```python
from build123d import *

# Parameters (mm, degrees)
SKETCH1_R           = 1.65
BOSS_EXTRUDE1_DEPTH = 22.4
SKETCH2_R           = 3.05
CUT_EXTRUDE1_DEPTH  = 3
CUT_EXTRUDE2_REACH  = 81.517
SKETCH3_W           = 0.4
SKETCH3_H           = 22.4


with BuildPart() as part:
    # Sketch1 → Boss-Extrude1 (new body)
    with BuildSketch(Plane.XY):
        Polygon((0, 0), (-75, 0), (-75, 7.5), (-0.787017068, 10), (72.903367057, 19.140247432), (74.076625545, 11.732584878), align=None)
        with Locations((-0.235377287, 2.990752001)):
            Circle(SKETCH1_R, mode=Mode.SUBTRACT)
    extrude(amount=BOSS_EXTRUDE1_DEPTH)

    # Sketch2 → Cut-Extrude1 (cut)
    with BuildSketch(Plane(origin=(0, 0, 0), x_dir=(0.9876883405951377, 0.15643446504023117, 0), z_dir=(0.1564344650402312, -0.9876883405951378, 0))):
        with Locations((67, 14.7)):
            Circle(SKETCH2_R)
        with Locations((67, 7.7)):
            Circle(SKETCH2_R)
    cut_extrude1 = extrude(amount=-CUT_EXTRUDE1_DEPTH, mode=Mode.SUBTRACT)

    # Mirror1: Cut-Extrude1 across plane
    add(cut_extrude1.mirror(Plane(origin=(0, 0, 0), x_dir=(0, 0, 1), z_dir=(0.9969173337331281, 0.07845909572784505, 0))), mode=Mode.SUBTRACT)

    # Cut-Extrude2: up to this plane
    cut_extrude2_end = Plane(origin=(-0.773549976, 9.600226767, 22.4), z_dir=(0.03366773042207346, -0.9994330812656876, 0))
    # Sketch3 → Cut-Extrude2 (cut, up to the surface)
    with BuildSketch(Plane(origin=(-1.048316472, 13.320123716, 0), x_dir=(0.9969173337331281, 0.07845909572784511, 0), z_dir=(-0.07845909572784511, 0.9969173337331281, 0)), mode=Mode.PRIVATE) as cut_extrude2_sk1:
        with Locations((0, -11.2)):
            Rectangle(SKETCH3_W, SKETCH3_H)
    cut_extrude2_tool1 = split(extrude(cut_extrude2_sk1.sketch, amount=-CUT_EXTRUDE2_REACH, mode=Mode.PRIVATE), bisect_by=cut_extrude2_end, keep=Keep.BOTH, mode=Mode.PRIVATE)
    add(cut_extrude2_tool1.solids().sort_by_distance((-1.048316, 13.320124, 11.2))[0], mode=Mode.SUBTRACT)


solid = part.part
```
Read the model definition and answer for the solid it produces. Units are mm, in the model's axes. A direction names the side the tool comes from. Round coordinates to 2 decimals unless told otherwise and drop trailing zeros. Loops run counter-clockwise (first coordinate to the right, second up) from the corner with the lowest first, then second, coordinate; pieces in that order, holes last. Notation, with made-up numbers: (33.25, 41.25) -> (39.25, 41.25) arc R24 ccw to (39.25, 77.25) -> close; hole circle Ø8 at (22, -18). An arc over 180 degrees is marked (long way). One line per item, written item: value.
1) A cutting plane is placed at B-B (x = -67). Determine the outline of the cut face in (y, z), and give its area (3 significant figures).
Answer list:
outline: (0, 0) -> (7.77, 0) -> (7.77, 22.4) -> (0, 22.4) -> (0, 17.75) -> (3, 17.75) -> (3, 11.65) -> (0, 11.65) -> (0, 10.75) -> (3, 10.75) -> (3, 4.65) -> (0, 4.65) -> close
area: 137 mm²
2) A cutting plane is placed at C-C (z = 16.25). Determine the outline of the cut face in (x, y), and give its area (3 significant figures).
Answer list:
outline: (-75, 0) -> (-69.63, 0) -> (-69.63, 3) -> (-64.37, 3) -> (-64.37, 0) -> (0, 0) -> (63.58, 10.07) -> (63.11, 13.03) -> (68.3, 13.86) -> (68.77, 10.89) -> (74.08, 11.73) -> (72.9, 19.14) -> (-0.59, 10.02) -> (-0.56, 9.61) -> (-0.96, 9.59) -> (-0.99, 9.99) -> (-75, 7.5) -> close; hole circle Ø3.3 at (-0.24, 2.99)
area: 1,270 mm²
3) A cutting plane is placed at A-A (z = 7.7). Determine the outline of the cut face in (x, y), and give its area (3 significant figures).
Answer list:
outline: (-75, 0) -> (-70.05, 0) -> (-70.05, 3) -> (-63.95, 3) -> (-63.95, 0) -> (0, 0) -> (63.16, 10) -> (62.69, 12.97) -> (68.72, 13.92) -> (69.19, 10.96) -> (74.08, 11.73) -> (72.9, 19.14) -> (-0.59, 10.02) -> (-0.56, 9.61) -> (-0.96, 9.59) -> (-0.99, 9.99) -> (-75, 7.5) -> close; hole circle Ø3.3 at (-0.24, 2.99)
area: 1,260 mm²
4) For faces 1 (the face through (65.552, 11.88, 17.724)), 2 (the face through (-67, 3, 15)), determine the directions among +Z, -Z, +X, -X, +Y, -Y from which every point of the face is accessible in a straight line to the end or side of a thin tool.
Answer list:
face 1: none
face 2: -Y
5) The mould has two halves that part along Z. Classify faces 3 (the face through (1, 8, 22.4)), 4 (the face through (73.48, 15.49, 11.04)), 5 (the face through (-63.953, 1.479, 7.834)), 6 (the face through (-67, 3, 8)): pulls with the +Z half, pulls with the -Z half, needs draft (parallel to the pull), parting line crosses it, or undercut.
Answer list:
face 3: pulls with the +Z half
face 4: needs draft
face 5: undercut
face 6: undercut
6) Flat-ended cylindrical pins translate along their axes: P1, Ø2, axis at x = -30.5, z = 4, coming from the +Y side; P2, Ø2, axis at x = 9.5, z = 9.5, coming from the +Y side; P3, Ø6, axis at x = -51, y = 12, coming from the -Z side; P4, Ø8, axis at x = 38, z = 13, coming from the -Y side. Find the tip coordinate at first contact, or state that the pin passes through.
Answer list:
P1: stops at y = 9.03
P2: stops at y = 11.4
P3: passes through
P4: stops at y = 5.39
7) A cutting plane is placed at D-D (x = 56). Determine the outline of the cut face in (y, z), and give its area (3 significant figures).
Answer list:
outline: (8.87, 0) -> (17.04, 0) -> (17.04, 22.4) -> (8.87, 22.4) -> close
area: 183 mm²
8) Consider L1, parallel to Z at x = -67, y = 2.35; L2, parallel to Y at x = 60.5, z = 20; L3, parallel to Y at x = -37, z = 19.75. Determine where each line is inside the solid, lowest interval first. Write a range as [from, to].
Answer list:
L1: z = [0, 4.65], [10.75, 11.65], [17.75, 22.4]
L2: y = [9.58, 17.6]
L3: y = [0, 8.78]
